Geometry: final body of the model. Coordinates: model frame, mm. A direction names the side the tool comes from. Give positions to 0.01 mm unless a question says otherwise; leave off trailing zeros. Write each loop counter-clockwise with the first axis right and the second up, starting at its lowest first coordinate (ties: lowest second). Pieces come first, ordered by that corner, then holes.
from build123d import *

# Parameters (mm, degrees)
BOSS_EXTRUDE1_DEPTH                           = 22.225
SKETCH2_W                                     = 3.81
SKETCH2_H                                     = 3.81
CUT_EXTRUDE1_DEPTH                            = 108.059192156
CUT_EXTRUDE2_DEPTH                            = 108.059192156
FILLET1_R                                     = 2.54
CSK_FOR_1_4_FLAT_HEAD_MACHINE_SCREW1_AT_COUNT = 2
CSK_FOR_1_4_FLAT_HEAD_MACHINE_SCREW1_AT_PITCH = 69.85
CUT_EXTRUDE3_DEPTH                            = 106.732743864
FILLET2_R                                     = 2.54
CHAMFER1_SIZE                                 = 3.81


with BuildPart() as part:
    # Sketch1 → Boss-Extrude1 (new, symmetric)
    with BuildSketch(Plane(origin=(0, 0, 0), x_dir=(1, 0, 0), z_dir=(0, 1, 0))):
        Polygon((0, 0), (0, 101.6), (-6.35, 101.6), (-6.35, 4.7625), (-25.4, 4.7625), (-25.4, 0), align=None)
    extrude(amount=BOSS_EXTRUDE1_DEPTH, both=True)

    # Sketch2 → Cut-Extrude1 (cut, through all)
    with BuildSketch(Plane.XY):
        with Locations((-1.905, 20.32)):
            Rectangle(SKETCH2_W, SKETCH2_H)
        with Locations((-1.905, -20.32)):
            Rectangle(SKETCH2_W, SKETCH2_H)
    extrude(amount=-CUT_EXTRUDE1_DEPTH, mode=Mode.SUBTRACT)

    # Sketch3 → Cut-Extrude2 (cut, through all)
    with BuildSketch(Plane.XY):
        with BuildLine():
            Line((-12.83335, -19.1262), (-17.32915, -19.1262))
            ThreePointArc((-17.32915, -19.1262), (-20.58035, -15.875), (-17.32915, -12.6238))
            Line((-17.32915, -12.6238), (-12.83335, -12.6238))
            ThreePointArc((-12.83335, -12.6238), (-9.58215, -15.875), (-12.83335, -19.1262))
        make_face()
        with BuildLine():
            Line((-12.83335, 19.1262), (-17.32915, 19.1262))
            ThreePointArc((-17.32915, 19.1262), (-20.58035, 15.875), (-17.32915, 12.6238))
            Line((-17.32915, 12.6238), (-12.83335, 12.6238))
            ThreePointArc((-12.83335, 12.6238), (-9.58215, 15.875), (-12.83335, 19.1262))
        make_face()
    extrude(amount=-CUT_EXTRUDE2_DEPTH, mode=Mode.SUBTRACT)

    # Fillet1
    fillet1_edges = [part.edges().sort_by_distance(p)[0] for p in [
        (-25.4, 22.225, -2.38125),
        (-25.4, -22.225, -2.38125),
    ]]
    fillet(fillet1_edges, radius=FILLET1_R)

    # Sketch5 → CSK for 1/4 Flat Head Machine Screw1 (revolve, cut)
    with BuildSketch(Plane(origin=(-6.35, 0, -19.05), x_dir=(0, 0, 1), z_dir=(0, 1, 0))):
        Polygon((0, 0), (0, 6.35), (3.57124, 6.35), (3.57124, 3.806858607), (6.8804917, 0), align=None)
    csk_for_1_4_flat_head_machine_screw1 = revolve(axis=Axis((-12.7, 0, -19.05), (1, 0, 0)), mode=Mode.SUBTRACT)

    # CSK for 1/4 Flat Head Machine Screw1 at: CSK for 1/4 Flat Head Machine Screw1 ×2
    with Locations(*[(0, 0, -i * CSK_FOR_1_4_FLAT_HEAD_MACHINE_SCREW1_AT_PITCH) for i in range(1, CSK_FOR_1_4_FLAT_HEAD_MACHINE_SCREW1_AT_COUNT)]):
        add(csk_for_1_4_flat_head_machine_screw1, mode=Mode.SUBTRACT)

    # Sketch6 → Cut-Extrude3 (cut, through all)
    with BuildSketch(Plane.ZY.offset(6.35)):
        Polygon((-88.9, -22.225), (-101.6, -22.225), (-101.6, -9.525), align=None)
        Polygon((-101.6, 22.225), (-101.6, 9.525), (-88.9, 22.225), align=None)
    extrude(amount=-CUT_EXTRUDE3_DEPTH, mode=Mode.SUBTRACT)

    # Fillet2
    fillet2_edges = [part.edges().sort_by_distance(p)[0] for p in [
        (-6.35, -15.875, -95.25),
        (-6.35, 0, -101.6),
        (-6.35, 15.875, -95.25),
        (-3.175, 9.525, -101.6),
        (-3.175, -9.525, -101.6),
    ]]
    fillet(fillet2_edges, radius=FILLET2_R)

    # Chamfer1
    chamfer1_edges = [part.edges().sort_by_distance(p)[0] for p in [
        (0, 18.415, -46.355),
        (0, -18.415, -46.355),
    ]]
    chamfer(chamfer1_edges, length=CHAMFER1_SIZE - 0.0001)  # a hair under: the kernel refuses the full size


solid = part.part
Q1. Pin query (flat end, axial travel): P1, Ø1, axis at y = 3.5, z = -56, coming from the -X side; P2, Ø11.5, axis at y = 0, z = -19.05, coming from the -X side; P3, Ø3, axis at y = -16, z = -83, coming from the +X side; P4, Ø3, axis at y = -20.5, z = -46.5, coming from the +X side. Return the tip coordinate at first contact, or that it passes through.
Filled sheet:
P1: stops at x = -6.35
P2: stops at x = -5.05
P3: stops at x = 0
P4: stops at x = -3.81
Q2. Pull-direction query (Y, two-part tool) for faces 6 (the cylindrical face through (-1.88, 9.46, -101.4)), 7 (the cylindrical face through (-1.289, -0.157, -92.468)), 8 (the flat face through (0, 0, -50)); classes: released by +Y, released by -Y, zero draft, split by the parting line, or undercut.
Filled sheet:
face 6: released by +Y
face 7: undercut
face 8: zero draft
Q3. Access query for faces 1 (the flat face through (-2, 0, -101.6)), 2 (the flat face through (-15, 19.126, -2)), 3 (the flat face through (-3.81, 20, -46)), 4 (the conical face through (-2.781, -0.166, -92.675)), 5 (the flat face through (-3.81, -20, -46)). Directions: +Z, -Z, +X, -X, +Y, -Y. A direction counts if a zero-diameter tool reaches every point of the face in a straight line with its end or side. Return the directions, or none.
Filled sheet:
face 1: -Z, +X, -X, +Y, -Y
face 2: +Z, -Z
face 3: +Z, -Z, +X, +Y
face 4: -X
face 5: +Z, -Z, +X, -Y
Q4. Ray query, line 1 along Z through (x, y) = (-0.65, 0); line 2 along Z through (x, y) = (-19.75, -8); line 3 along Y through (x, z) = (-1.6, -88.9). Return the intervals inside material, ascending.
Filled sheet:
line 1: z = -101.6 to -92.47, -85.33 to -22.62, -15.48 to 0
line 2: z = -4.76 to 0
line 3: y = -16.21 to -3.57, 3.57 to 16.21
Q5. Section C-C on x = -15.25. Output: boundary loops of the cut face in (y, z) (1 decimal), plus the area to 3 significant figures.
Filled sheet:
outline: (-22.2, -4.8) - (-19.1, -4.8) - (-19.1, 0) - (-22.2, 0) - close; (-12.6, -4.8) - (12.6, -4.8) - (12.6, 0) - (-12.6, 0) - close; (19.1, -4.8) - (22.2, -4.8) - (22.2, 0) - (19.1, 0) - close
area: 150 mm2
Q6. Section B-B on y = 0. Output: boundary loops of the cut face in (x, z).
Filled sheet:
outline: (-25.4, -4.76) - (-6.35, -4.76) - (-6.35, -12.17) - (-2.54, -15.48) - (0, -15.48) - (0, 0) - (-25.4, 0) - close; (-6.35, -99.06) arc R2.54 ccw to (-3.81, -101.6) - (0, -101.6) - (0, -92.47) - (-2.54, -92.47) - (-6.35, -95.78) - close; (-6.35, -82.02) - (-2.54, -85.33) - (0, -85.33) - (0, -22.62) - (-2.54, -22.62) - (-6.35, -25.93) - close
